Model file for the job. Use its own axes, mm. Give positions to 0.01 mm unless a question says otherwise; leave off trailing zeros. Loops run counter-clockwise (first coordinate to the right, second up) from the corner with the lowest first, then second, coordinate; pieces in that order, holes last. Notation, with made-up numbers: (25.25, -35.5) -> (70.25, -35.5) arc R20 cw to (70.25, -25.5) -> close; hole circle Ø6 at (70.5, 33.5). An arc over 180 degrees is marked (long way). Use CSV: the item, a comma, the result in double quotes. Start each with the question number.
(1) Cut at A-A on z = 374.65. Write the cut outline in (x, y).
(2) Flat gauge pins, fed straight in: pin 1 (6.5 mm diameter, centred on y = 0, z = 6.35, fed in from -X); pin 2 (1.5 mm diameter, centred on x = 1, z = 49.5, fed in from -Y). Where does each tip first touch, or does it go through?
(3) Cut at B-B on z = 52. Write the cut outline in (x, y) (3 decimals), then the cut area to 3 significant figures.
(4) Pull direction Y, two halves, no side cores. Call faces 1 (the flat face through (-3.219, -5.474, 187.833)), 2 (the flat face through (6.35, 0, 188)), 3 (the cylindrical face through (-3.8, -1.92, 377.66)): pulls with the +Y half, pulls with the -Y half, needs draft (parallel to the pull), parting line crosses it, or undercut.
(5) Drill centre lines: probe 1 along Z at (x, y) = (-5, 0); probe 2 along Z at (x, y) = (4.25, 0.5); probe 3 along X at (y, z) = (-0.5, 26) (3 decimals). Where is each one in solid material? Low to high.
from build123d import *

# Parameters (mm, degrees)
F1_DEPTH = 381
F3_D     = 7.1374
F5_D     = 3.7973
F5_DEPTH = 9.53516
F5_TIP   = 1.1408240143


with BuildPart() as f1:
    # F0 (on Top) → F1 (new body)
    with BuildSketch(Plane.XY):
        Polygon((6.35, 3.6661742094), (0, 7.3323484187), (-6.35, 3.6661742094), (-6.35, -3.6661742094), (0, -7.3323484187), (6.35, -3.6661742094), align=None)
        Polygon((0, 3.6661742094), (3.175, 1.8330871047), (3.175, -1.8330871047), (0, -3.6661742094), (-3.175, -1.8330871047), (-3.175, 1.8330871047), align=None, mode=Mode.SUBTRACT)
    extrude(amount=F1_DEPTH)

    # F3 (through all)
    with Locations(Plane.YZ.offset(6.35)):
        with Locations((0, 374.65), (0, 6.35)):
            Hole(F3_D / 2)

    # F5
    with Locations(Plane(origin=(-6.35, 0, 0), x_dir=(0, -1, 0), z_dir=(-1, 0, 0))):
        with Locations((0, 279.4)):
            Hole(F5_D / 2, depth=F5_DEPTH)
            with Locations((0, 0, -(F5_DEPTH + F5_TIP / 2))):  # 118° drill point
                Cone(0, F5_D / 2, F5_TIP, mode=Mode.SUBTRACT)


solid = f1.part
Check result:
1,outline,"(-6.35, -3.67) -> (0, -7.33) -> (6.35, -3.67) -> (6.35, -3.57) -> (0.17, -3.57) -> (0, -3.67) -> (-0.17, -3.57) -> (-6.35, -3.57) -> close; (-6.35, 3.57) -> (-0.17, 3.57) -> (0, 3.67) -> (0.17, 3.57) -> (6.35, 3.57) -> (6.35, 3.67) -> (0, 7.33) -> (-6.35, 3.67) -> close"
2,pin 1,"through"
2,pin 2,"y = -7.19"
3,outline,"(-6.35, -3.666) -> (0, -7.332) -> (6.35, -3.666) -> (6.35, 3.666) -> (0, 7.332) -> (-6.35, 3.666) -> close; hole (-3.175, -1.833) -> (0, -3.666) -> (3.175, -1.833) -> (3.175, 1.833) -> (0, 3.666) -> (-3.175, 1.833) -> close"
3,area,"105 mm²"
4,face 1,"pulls with the -Y half"
4,face 2,"needs draft"
4,face 3,"undercut"
5,probe 1,"0 to 2.78, 9.92 to 277.5, 281.3 to 371.08, 378.22 to 381"
5,probe 2,"0 to 2.82, 9.88 to 371.12, 378.18 to 381"
5,probe 3,"-6.35 to -3.175, 3.175 to 6.35"
